Part model, mm, in its own coordinate system. A direction names the side the tool comes from. Round coordinates to 2 decimals unless told otherwise and drop trailing zeros. Loops run counter-clockwise (first coordinate to the right, second up) from the corner with the lowest first, then second, coordinate; pieces in that order, holes last.
(1) Cut at A-A on z = 0. List the corners of the cut face in (x, y).
(2) Flat gauge pins, fed straight in: pin 1 (1 mm diameter, centred on y = -3, z = -22.5, fed in from +X); pin 2 (10 mm diameter, centred on y = 9.5, z = 1, fed in from +X); pin 3 (3 mm diameter, centred on y = 5.5, z = 25, fed in from -X); pin 4 (3 mm diameter, centred on x = 6.5, z = 8.5, fed in from +Y). Where does each tip first touch, or does it go through?
(3) Cut at C-C on x = 10.5. List the corners of the cut face in (y, z), then the cut area to 3 significant figures.
(4) Probe probe 1 along Y at (x, z) = (-8.5, 0); probe 2 along Y at (x, z) = (-1, 0); probe 3 along X at (y, z) = (43, -0.5). List the from-to ranges inside material, lowest first.
(5) Mould opens along X. For faces 6 (the face through (18, -15, 4)), 7 (the face through (3.25, 35.08, 7.79)), 8 (the face through (0.042, 34.168, 7.587)), 9 (the face through (-9.96, -15.02, -47.69)) say: +X half, -X half, draft (parallel to the pull), parting line (faces both ways), or undercut.
(6) Tool access for faces 1 (the face through (-13, 22, 10)), 2 (the face through (13, 22, -10)), 3 (the face through (-3.194, -10.732, -34.078)), 4 (the face through (-18, -15, -4)), 5 (the face through (10.04, -15.02, -47.69)): list every direction of +Z, -Z, +X, -X, +Y, -Y with a clear straight run to the whole face (end or side of a thin tool).
from build123d import *


with BuildPart() as part:
    # Sketch1 → Revolve1 (revolve)
    with BuildSketch(Plane.XY, mode=Mode.PRIVATE) as revolve1_sk:
        with BuildLine():
            Line((18, 15), (-18, 15))
            Line((-18, 15), (-18, 18))
            ThreePointArc((-18, 18), (-14.538750305, 18.798437881), (-13, 22))
            Line((-13, 22), (-13, 50))
            Line((-13, 50), (-7, 50))
            Line((-7, 50), (-3, 35))
            Line((-3, 35), (3, 35))
            Line((3, 35), (7, 50))
            Line((7, 50), (13, 50))
            Line((13, 50), (13, 22))
            ThreePointArc((13, 22), (14.538750305, 18.798437881), (18, 18))
            Line((18, 18), (18, 15))
        make_face()
    revolve(revolve1_sk.sketch.rotate(Axis((38.229944377, 0, 0), (-1, 0, 0)), 90), axis=Axis((38.229944377, 0, 0), (-1, 0, 0)))


solid = part.part
Final values:
1. outline: (-18, -18) arc R4.1 cw to (-13, -22) - (-13, -50) - (-7, -50) - (-3, -35) - (3, -35) - (7, -50) - (13, -50) - (13, -22) arc R4.1 cw to (18, -18) - (18, -15) - (-18, -15) - close; (-18, 15) - (18, 15) - (18, 18) arc R4.1 cw to (13, 22) - (13, 50) - (7, 50) - (3, 35) - (-3, 35) - (-7, 50) - (-13, 50) - (-13, 22) arc R4.1 cw to (-18, 18) - close
2. pin 1: stops at x = 13
2. pin 2: passes through
2. pin 3: stops at x = -13
2. pin 4: stops at y = 49.5
3. outline: circle Ø100 at (0, 0); hole circle Ø30 at (0, 0)
3. area: 7,150 mm2
4. probe 1: y = -50 to -15, 15 to 50
4. probe 2: y = -35 to -15, 15 to 35
4. probe 3: x = -13 to -5.13, 5.13 to 13
5. face 6: +X half
5. face 7: undercut
5. face 8: undercut
5. face 9: draft
6. face 1: -X
6. face 2: +X
6. face 3: none
6. face 4: +Z, -Z, -X, +Y, -Y
6. face 5: +X, -X
